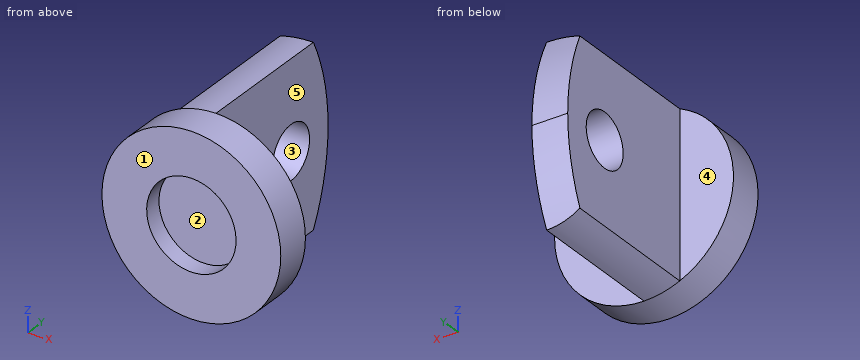
```python
from build123d import *

# Parameters (mm, degrees)
BOSS_EXTRUDE1_START = 455
BOSS_EXTRUDE1_DEPTH = 455
SKETCH4_R           = 75
CUT_EXTRUDE1_DEPTH  = 100


with BuildPart() as part:
    # Sketch1 → Revolve1 (revolve)
    with BuildSketch(Plane.XY, mode=Mode.PRIVATE) as revolve1_sk:
        Polygon((0, 50), (125, 50), (125, 0), (250, 0), (250, 100), (0, 100), align=None)
    revolve(revolve1_sk.sketch.rotate(Axis((0, 188.75, 0), (0, -1, 0)), 90), axis=Axis((0, 188.75, 0), (0, -1, 0)))

    # Sketch3 → Boss-Extrude1 (add)
    with BuildSketch(Plane(origin=(0, 100, 0), x_dir=(1, 0, 0), z_dir=(0, 1, 0)).offset(BOSS_EXTRUDE1_START)):
        with BuildLine():
            Line((0, 250), (0, -250))
            ThreePointArc((0, -250), (-51.077410922, -244.726578233), (-100, -229.128784748))
            Line((-100, -229.128784748), (-100, 229.128784748))
            ThreePointArc((-100, 229.128784748), (-51.077410922, 244.726578233), (0, 250))
        make_face()
    extrude(amount=-BOSS_EXTRUDE1_DEPTH)

    # Sketch4 → Cut-Extrude1 (cut)
    with BuildSketch(Plane(origin=(0, 0, 0), x_dir=(0, 0, -1), z_dir=(1, 0, 0))):
        with Locations((0, 405)):
            Circle(SKETCH4_R)
        with BuildLine():
            Line((-250, 555), (-250, 495.504793115))
            ThreePointArc((-250, 495.504793115), (-128.490932522, 539.921364885), (1.363e-06, 555))
            Line((1.363e-06, 555), (-250, 555))
        make_face()
        with BuildLine():
            Line((250, 555), (1.363e-06, 555))
            ThreePointArc((1.363e-06, 555), (128.490933847, 539.92136457), (250, 495.504793115))
            Line((250, 495.504793115), (250, 555))
        make_face()
    extrude(amount=-CUT_EXTRUDE1_DEPTH, mode=Mode.SUBTRACT)


solid = part.part
```
Verification items for the finished model (mm, model axes). Face numbers are marked on the shaded views. A direction names the side the tool comes from. Round coordinates to 2 decimals unless told otherwise and drop trailing zeros. Write each loop counter-clockwise with the first axis right and the second up, starting at its lowest first coordinate (ties: lowest second). Pieces come first, ordered by that corner, then holes. Notation, with made-up numbers: (48.25, 38) -> (79.25, 38) arc R18 cw to (79.25, 67) -> close; hole circle Ø5 at (-6, 33). An arc over 180 degrees is marked (long way). Write each question's results on one line, items separated by ' | '. Start each with the question number.
1. Depth check by flat-ended pin: P1, Ø3, axis at x = 146, z = -144, coming from the -Y side; P2, Ø10, axis at x = -90.5, y = 309, coming from the -Z side (3 decimals); P3, Ø2, axis at y = 153.5, z = -164.5, coming from the +X side; P4, Ø12, axis at x = -59, z = 186.5, coming from the +Y side. Enter the tip coordinate at first touch or a pass-through.
2. Set-up check for the marked faces 3, 4 and 5: record each of +Z, -Z, +X, -X, +Y, -Y from which the full face is reachable in a straight line by a thin tool's end or side.
3. Cross-section at C-C (z = 64). Enter the section's corners in (x, y), then the cut area to 3 significant figures.
4. Material ranges on probe 1 along X at (y, z) = (27, 0); probe 2 along Y at (x, z) = (81.5, 194); probe 3 along X at (y, z) = (461, -143.5), recorded low to high. Write a range as from..to.
5. Cross-section at B-B (x = -16). Enter the section's corners in (y, z), then the cut area to 3 significant figures.
6. Cross-section at A-A (y = 405). Enter the section's corners in (x, z), then the cut area to 3 significant figures.
7. Cross-section at D-D (x = 59). Enter the section's corners in (y, z).
8. Draft check along Z on the marked faces 1 and 2. Enter one of: +Z half, -Z half, draft (parallel to the pull), parting line (faces both ways), or undercut.
Solutions:
1) P1: stops at y = 0 | P2: stops at z = -234.925 | P3: stops at x = 0 | P4: stops at y = 524.83
2) face 3: +X, -X | face 4: +Z, -Z, -X, +Y | face 5: +Z, -Z, +X, +Y
3) outline: (-241.67, 0) -> (-107.37, 0) -> (-107.37, 50) -> (107.37, 50) -> (107.37, 0) -> (241.67, 0) -> (241.67, 100) -> (0, 100) -> (0, 365.9) -> (-100, 365.9) -> (-100, 100) -> (-241.67, 100) -> close; (-100, 444.1) -> (0, 444.1) -> (0, 551.3) -> (-100, 551.3) -> close | area: 74,900 mm2
4) probe 1: x = -250..-125, 125..250 | probe 2: y = 0..100 | probe 3: x = -100..0
5) outline: (0, -249.49) -> (495.76, -249.49) arc R555 ccw to (495.76, 249.49) -> (0, 249.49) -> (0, 123.97) -> (50, 123.97) -> (50, -123.97) -> (0, -123.97) -> close; hole circle Ø150 at (405, 0) | area: 237,000 mm2
6) outline: (-100, -229.13) arc R250 ccw to (0, -250) -> (0, -75) -> (-100, -75) -> close; (-100, 75) -> (0, 75) -> (0, 250) arc R250 ccw to (-100, 229.13) -> close | area: 33,600 mm2
7) outline: (0, -242.94) -> (100, -242.94) -> (100, 242.94) -> (0, 242.94) -> (0, 110.2) -> (50, 110.2) -> (50, -110.2) -> (0, -110.2) -> close
8) face 1: draft | face 2: undercut
